Verification items for the finished model (mm, model axes). A direction names the side the tool comes from. Coordinates: 2 decimals unless noted, no trailing zeros. Order: outer loops, then holes, each group sorted by start corner. A loop starts at its lowest first (then second) coordinate and runs counter-clockwise, first axis right, second up. Notation, with made-up numbers: (-26, 43.25) -> (31, 43.25) arc R19 cw to (31, 47.25) -> close; hole circle Ø6 at (-29.5, 0.25). An arc over 180 degrees is marked (long way). Answer as CSV lines item,"result".
```python
from build123d import *

# Parameters (mm, degrees)
SKETCH_1_W          = 30
SKETCH_1_H          = 23
EXTRUDE_1_DEPTH     = 72
SKETCH_2_W          = 27
SKETCH_2_H          = 20
CUT_EXTRUDE_1_DEPTH = 20
SKETCH_3_R          = 4.1
CUT_EXTRUDE_2_DEPTH = 6
SKETCH_7_W          = 15
SKETCH_7_H          = 10
EXTRUDE_2_DEPTH     = 23
EXTRUDE_3_DEPTH     = 20
EXTRUDE_START       = 6
SKETCH_11_R         = 4.1
EXTRUDE_5_DEPTH     = 6
SKETCH_12_R         = 1.45
CUT_EXTRUDE_3_DEPTH = 5
SKETCH_13_R         = 1.45
CUT_EXTRUDE_4_DEPTH = 1.5
SKETCH_14_W         = 7.1
SKETCH_14_H         = 0.1
SKETCH_14_W_2       = 14.1
SKETCH_14_W_3       = 0.1
SKETCH_14_H_2       = 13.1
CUT_EXTRUDE_5_DEPTH = 20
EXTRUDE_6_DEPTH     = 6.6


with BuildPart() as part:
    # 草图1 → 凸台-拉伸1 (new body)
    with BuildSketch(Plane(origin=(0, 0, 0), x_dir=(1, 0, 0), z_dir=(0, 1, 0))):
        with Locations((15, 11.5)):
            Rectangle(SKETCH_1_W, SKETCH_1_H)
    extrude(amount=EXTRUDE_1_DEPTH)

    # 草图2 → 切除-拉伸1 (cut)
    with BuildSketch(Plane.XZ):
        with Locations((16.5, -10)):
            Rectangle(SKETCH_2_W, SKETCH_2_H)
    extrude(amount=-CUT_EXTRUDE_1_DEPTH, mode=Mode.SUBTRACT)

    # 草图3 → 切除-拉伸2 (cut)
    with BuildSketch(Plane.XY):
        with Locations((13, 40)):
            Circle(SKETCH_3_R)
    extrude(amount=-CUT_EXTRUDE_2_DEPTH, mode=Mode.SUBTRACT)

    # 草图7 → 凸台-拉伸2 (add)
    with BuildSketch(Plane(origin=(0, 0, -23), x_dir=(-1, 0, 0), z_dir=(0, 0, -1))):
        with Locations((-37.5, 67)):
            Rectangle(SKETCH_7_W, SKETCH_7_H)
    extrude(amount=-EXTRUDE_2_DEPTH)

    # 草图9 → 凸台-拉伸3 (add)
    with BuildSketch(Plane.XZ.offset(-20)):
        Polygon((10.1, -20), (15.9, -20), (15.9, -18.3), (18.3, -18.3), (18.3, -16.732842713), (15.667157288, -14.1), (10.332842713, -14.1), (7.7, -16.732842713), (7.7, -18.3), (10.1, -18.3), align=None)
    extrude_3 = extrude(amount=EXTRUDE_3_DEPTH)

    # 镜向1: 凸台-拉伸3 across plane
    add(extrude_3.mirror(Plane(origin=(11.5, 0, -11.5), x_dir=(0.7071067811865478, 0, 0.7071067811865472), z_dir=(0.7071067811865475, 0, -0.7071067811865477))))

    # 草图11 → 凸台-拉伸5 (add)
    with BuildSketch(Plane.XY.offset(EXTRUDE_START)):
        Polygon((0, 0), (3, 0), (3, 20), (30, 20), (30, 62), (45, 62), (45, 72), (0, 72), align=None)
        with Locations((13, 40)):
            Circle(SKETCH_11_R, mode=Mode.SUBTRACT)
    extrude(amount=-EXTRUDE_5_DEPTH)

    # 草图12 → 切除-拉伸3 (cut)
    with BuildSketch(Plane(origin=(0, 72, 0), x_dir=(1, 0, 0), z_dir=(0, 1, 0))):
        with Locations(Location((21, 14, 0), (0, 0, 270))):
            Circle(SKETCH_12_R)
        with Locations(Location((36, -1, 0), (0, 0, 270))):
            Circle(SKETCH_12_R)
    extrude(amount=-CUT_EXTRUDE_3_DEPTH, mode=Mode.SUBTRACT)

    # 草图13 → 切除-拉伸4 (cut)
    with BuildSketch(Plane(origin=(0, 67, 0), x_dir=(1, 0, 0), z_dir=(0, 1, 0))):
        with Locations(Location((21, 14, 0), (0, 0, 270))):
            Circle(SKETCH_13_R)
    extrude(amount=-CUT_EXTRUDE_4_DEPTH, mode=Mode.SUBTRACT)

    # 草图14 → 切除-拉伸5 (cut)
    with BuildSketch(Plane.XZ):
        with Locations((6.55, -20.05)):
            Rectangle(SKETCH_14_W, SKETCH_14_H)
        Polygon((3, -12.9), (2.9, -12.9), (2.9, -20.1), (3, -20.1), (3, -20), align=None)
        with Locations((22.95, -20.05)):
            Rectangle(SKETCH_14_W_2, SKETCH_14_H)
        with Locations((2.95, -0.55)):
            Rectangle(SKETCH_14_W_3, SKETCH_14_H_2)
    extrude(amount=-CUT_EXTRUDE_5_DEPTH, mode=Mode.SUBTRACT)

    # 草图15 → 凸台-拉伸6 (add)
    with BuildSketch(Plane.XZ):
        Polygon((4.7, -7.1), (2.9, -7.1), (2.9, 6), (0, 6), (0, -23), (30, -23), (30, -20.1), (15.9, -20.1), (15.9, -18.3), (18.3, -18.3), (18.3, -16.732842713), (15.667157288, -14.1), (10.332842713, -14.1), (7.7, -16.732842713), (7.7, -18.3), (10.1, -18.3), (10.1, -20.1), (2.9, -20.1), (2.9, -12.9), (4.7, -12.9), (4.7, -15.3), (6.267157287, -15.3), (8.9, -12.667157287), (8.9, -7.332842712), (6.267157287, -4.7), (4.7, -4.7), align=None)
    extrude(amount=EXTRUDE_6_DEPTH)


solid = part.part
```
Item 1: Section check B-B, the plane y = 40. Record the boundary of the cut face in (x, z), plus the area to 3 significant figures.
Answer list:
outline,"(0, -23) -> (30, -23) -> (30, 6) -> (17.1, 6) -> (17.1, -6) -> (8.9, -6) -> (8.9, 6) -> (0, 6) -> close"
area,"772 mm2"
Item 2: Section check C-C, the plane x = 36. Record the boundary of the cut face in (y, z).
Answer list:
outline,"(62, -23) -> (72, -23) -> (72, -0.45) -> (67, -0.45) -> (67, 2.45) -> (72, 2.45) -> (72, 6) -> (62, 6) -> close"
Item 3: Section check A-A, the plane z = 1. Record the boundary of the cut face in (x, y), plus the area to 3 significant figures.
Answer list:
outline,"(0, -6.6) -> (2.9, -6.6) -> (2.9, 20) -> (30, 20) -> (30, 62) -> (45, 62) -> (45, 72) -> (37.45, 72) -> (37.45, 67) -> (34.55, 67) -> (34.55, 72) -> (0, 72) -> close; hole circle Ø8.2 at (13, 40)"
area,"1,720 mm2"
Item 4: Release check for a two-part mould opening along X. For faces 1 (the flat face through (30, 36, -9)), 2 (the flat face through (23, 7, -20.1)), 3 (the flat face through (4.7, 7, -14)), 4 (the flat face through (36, 67, 1)) record: +X half, -X half, draft (parallel to the pull), parting line (faces both ways), or undercut.
Answer list:
face 1,"+X half"
face 2,"draft"
face 3,"undercut"
face 4,"undercut"
Item 5: Depth check by flat-ended pin: pin 1 Ø4 at (x, y) = (14, 39.5) entering from +Z; pin 2 Ø1.7 at (x, z) = (21, -14) entering from -Y; pin 3 Ø0.9 at (x, z) = (36.5, 1.5) entering from +Y. Enter the tip coordinate at first touch or a pass-through.
Answer list:
pin 1,"z = -6"
pin 2,"y = 20"
pin 3,"y = 67"
Item 6: Thickness scan on line 1 (X direction, y = 70, z = -14); line 2 (Y direction, x = 13, z = 3); line 3 (Y direction, x = 29, z = -7.25). Record the ranges inside material, lowest first.
Answer list:
line 1,"0 to 19.55, 22.45 to 45"
line 2,"20 to 35.9, 44.1 to 72"
line 3,"20 to 72"
Item 7: Tool access check on faces 5 (the flat face through (5, 7, -4.7)), 6 (the flat face through (10.1, 7, -19)), 7 (the flat face through (21, 65.5, -14)), 8 (the flat face through (37, 62, -8)). Record the directions out of +Z, -Z, +X, -X, +Y, -Y that give a thin tool (end or side, any length) a straight path to the whole face; none if there is none.
Answer list:
face 5,"+Z, +X, -Y"
face 6,"-Y"
face 7,"+Y"
face 8,"+Z, -Z, +X, -Y"
Item 8: Section check D-D, the plane y = 4. Record the boundary of the cut face in (x, z), plus the area to 3 significant figures.
Answer list:
outline,"(0, -23) -> (30, -23) -> (30, -20.1) -> (15.9, -20.1) -> (15.9, -18.3) -> (18.3, -18.3) -> (18.3, -16.73) -> (15.67, -14.1) -> (10.33, -14.1) -> (7.7, -16.73) -> (7.7, -18.3) -> (10.1, -18.3) -> (10.1, -20.1) -> (2.9, -20.1) -> (2.9, -12.9) -> (4.7, -12.9) -> (4.7, -15.3) -> (6.27, -15.3) -> (8.9, -12.67) -> (8.9, -7.33) -> (6.27, -4.7) -> (4.7, -4.7) -> (4.7, -7.1) -> (2.9, -7.1) -> (2.9, 6) -> (0, 6) -> close"
area,"259 mm2"
